Answer from the drawing. Dimensions are ordinates in mm from the lowest x, y and z of the part. Give positions to 0.01 mm unless a question says otherwise; leave off trailing zeros. Order: outer loops, then holes, each group sorted by start corner. A loop starts at its lowest first (then second) coordinate and runs counter-clockwise, first axis right, second up.
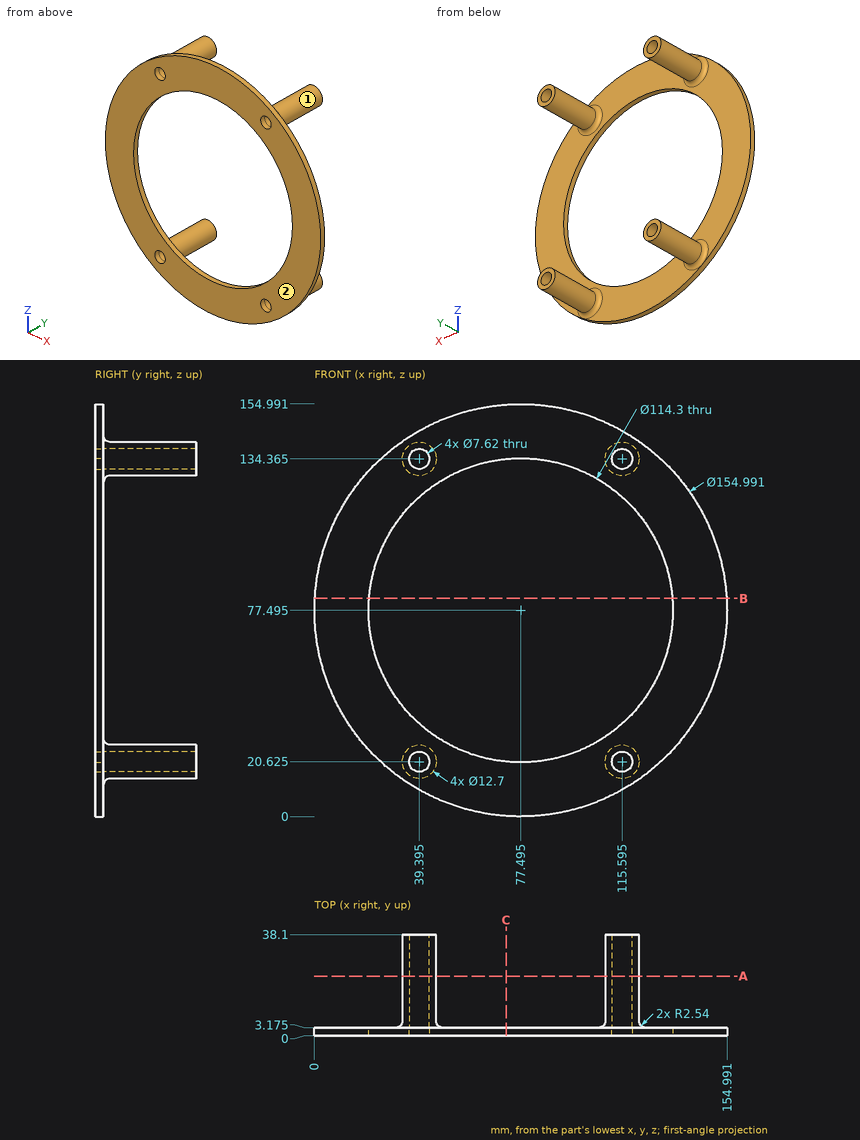
1. The part is cut by section C-C (x = 72). Write down the section's boundary in (y, z) (1 decimal).
Findings below:
outline: (0, 0.2) - (3.2, 0.2) - (3.2, 20.6) - (0, 20.6) - close; (0, 134.4) - (3.2, 134.4) - (3.2, 154.8) - (0, 154.8) - close
2. The mould has two halves that part along X. Classify the marked faces 1 and 2: pulls with the +X half, pulls with the -X half, needs draft (parallel to the pull), parting line crosses it, or undercut.
Findings below:
face 1: undercut
face 2: needs draft
3. Straight lines are drawn through the part: probe 1 along X at (y, z) = (15, 24) (1 decimal); probe 2 along Y at (x, z) = (60, 9) (1 decimal); probe 3 along X at (y, z) = (3, 73). For each, find the intervals that lie inside material, in ascending order.
Findings below:
probe 1: x = 34 to 37.6, 41.2 to 44.8, 110.2 to 113.8, 117.4 to 121
probe 2: y = 0 to 3.2
probe 3: x = 0.13 to 20.52, 134.47 to 154.86
4. Given P1, Ø4, axis at y = 18.5, z = 136.5, coming from the +X side; P2, Ø7, axis at x = 115.6, z = 134.37, coming from the -Y side; P3, Ø8, axis at x = 44, z = 124, coming from the +Y side; P4, Ø8, axis at x = 33.5, y = 29.5, coming from the +Z side, each flat-ended and moving along its own axis, determine where each tip first touches the part or whether it passes through.
Findings below:
P1: stops at x = 121.94
P2: passes through
P3: stops at y = 3.7
P4: stops at z = 140.43
5. The part is cut by section A-A (y = 22.5). State how many separate pieces and enclosed holes the cut face has.
Findings below:
separate pieces: 4
enclosed holes: 4
6. The part is cut by section B-B (z = 82). Write down the section's boundary in (x, y) (1 decimal).
Findings below:
outline: (0.1, 0) - (20.5, 0) - (20.5, 3.2) - (0.1, 3.2) - close; (134.5, 0) - (154.9, 0) - (154.9, 3.2) - (134.5, 3.2) - close
